Study the drawing (mm; zero at the part's minimum x, y, z) and answer. A direction names the side the tool comes from. Round coordinates to 2 decimals unless told otherwise and drop trailing zeros. Write each loop counter-clockwise with the first axis right and the second up, starting at its lowest first coordinate (ties: lowest second). Pieces come first, ordered by that corner, then holes. Notation, with made-up numbers: (26, -3) - (64, -3) arc R11 ccw to (64, 11) - close; hole circle Ø8 at (-35.5, -5). An arc over 180 degrees is marked (long way). Return JSON: item names as keys, results as strings. Group by question number.
(1) Which of the six approach directions +Z, -Z, +X, -X, +Y, -Y give full straight-line access (tool end or side, diameter ignored) to the marked faces 1, 2 and 3?
(2) Section D-D, the plane z = 12.25 is taken. Write down the section's boundary in (x, y).
(3) Section C-C, the plane y = 0.35 is taken. Write down the section's boundary in (x, z).
(4) Find the intervals of material crossed by line 1 along X through (y, z) = (0.6, 7.25); line 2 along Z through (x, y) = (18.5, 1.9); line 3 along Z through (x, y) = (31, 2.8), in increasing order. Write a range as [from, to].
(5) Each of these flat-tipped pins is pushed along its axis until it touches: pin 1 (0.9 mm diameter, centred on x = 8, y = 2, fed in from +Z); pin 2 (1 mm diameter, centred on y = 2.5, z = 10.5, fed in from -X); pin 3 (1 mm diameter, centred on x = 23.5, y = 1.5, fed in from -Z); pin 4 (1.5 mm diameter, centred on x = 3.5, y = 1.5, fed in from -Z). Where does it stop, or does it pass through?
(6) Determine the mould class of the marked faces 4, 5, 6 and 7 for opening direction X: +X half, -X half, draft (parallel to the pull), parting line (faces both ways), or undercut.
(7) Section B-B, the plane z = 7.25 is taken. Write down the section's boundary in (x, y).
(8) Section A-A, the plane x = 18.35 is taken. Write down the section's boundary in (y, z).
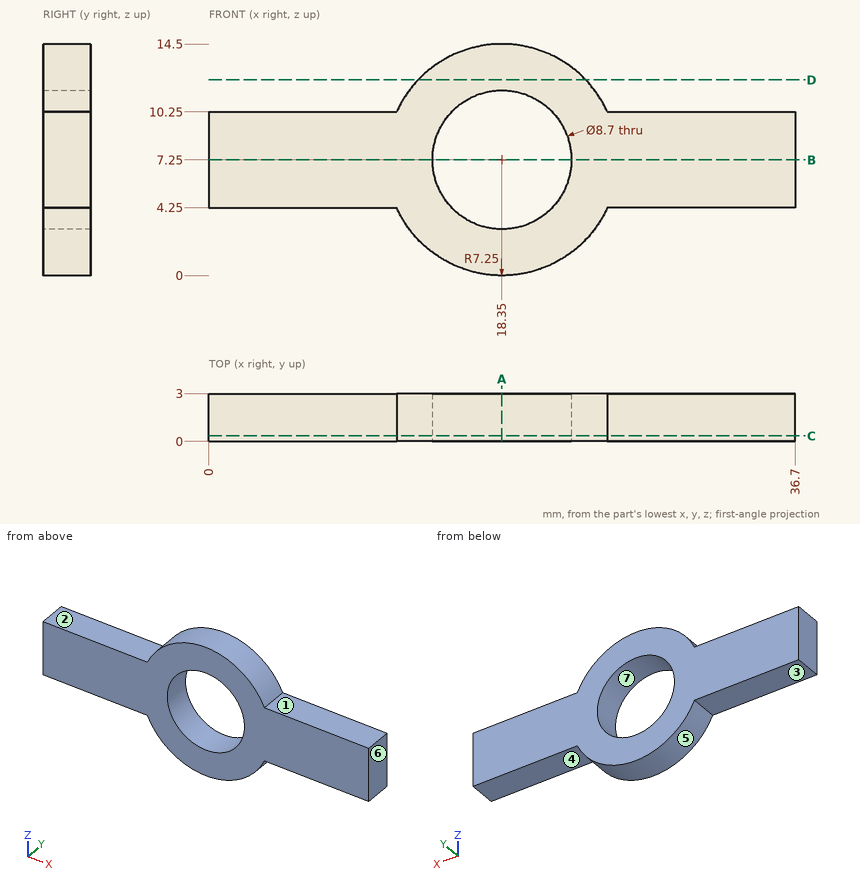
Working result:
{
 "1": {"face 1": "+Z, +X, +Y, -Y", "face 2": "+Z, -X, +Y, -Y", "face 3": "-Z, -X, +Y, -Y"},
 "2": {"outline": "(13.1, 0) - (23.6, 0) - (23.6, 3) - (13.1, 3) - close"},
 "3": {"outline": "(0, 4.25) - (11.75, 4.25) arc R7.25 ccw to (24.95, 4.25) - (36.7, 4.25) - (36.7, 10.25) - (24.95, 10.25) arc R7.25 ccw to (11.75, 10.25) - (0, 10.25) - close; hole circle Ø8.7 at (18.35, 7.25)"},
 "4": {"line 1": "x = [0, 14], [22.7, 36.7]", "line 2": "z = [0, 2.9], [11.6, 14.5]", "line 3": "z = [4.25, 10.25]"},
 "5": {"pin 1": "stops at z = 10.25", "pin 2": "stops at x = 0", "pin 3": "stops at z = 1.69", "pin 4": "stops at z = 4.25"},
 "6": {"face 4": "draft", "face 5": "parting line", "face 6": "+X half", "face 7": "undercut"},
 "7": {"outline": "(0, 0) - (14, 0) - (14, 3) - (0, 3) - close; (22.7, 0) - (36.7, 0) - (36.7, 3) - (22.7, 3) - close"},
 "8": {"outline": "(0, 0) - (3, 0) - (3, 2.9) - (0, 2.9) - close; (0, 11.6) - (3, 11.6) - (3, 14.5) - (0, 14.5) - close"}
}
